Autodesk Inventor part; units mm, degrees
ref_plane "YZ Plane" through (0, 0, 0) normal (1, 0, 0) x (0, 1, 0)
ref_plane "XZ Plane" through (0, 0, 0) normal (0, 1, 0) x (-1, 0, 0)
ref_plane "XY Plane" through (0, 0, 0) normal (0, 0, 1) x (1, 0, 0)
sketch "Sketch1" plane through (0, 0, 0) normal (0, 0, 1) x (1, 0, 0)
  line L0 (0, 0) -> (25.4, 0)
  line L1 (25.4, 0) -> (25.4, -50.8)
  line L2 (25.4, -50.8) -> (0, -50.8)
  line L3 (0, -50.8) -> (0, 0)
  line L4 (3.175, -3.175) -> (22.225, -3.175)
  line L5 (22.225, -3.175) -> (22.225, -47.625)
  line L6 (22.225, -47.625) -> (3.175, -47.625)
  line L7 (3.175, -47.625) -> (3.175, -3.175)
  dimension "d0" = 25.4
  dimension "d1" = 50.8
  dimension "d2" = 19.05
  dimension "d3" = 44.45
  dimension "d4" = 3.175
  dimension "d5" = 3.175
extrude "Extrusion1" add sketch "Sketch1" along normal blind 76.2
sketch "Sketch2" plane through (0, -50.8, 0) normal (-1, 0, 0) x (0, 0, 1)
  line L0 (0, 0) -> (0, 50.8)
  line L1 (0, 0) -> (76.2, 0)
  point P0 (25.4, 20.6375)
  dimension "d8" = 20.6375
  dimension "d9" = 25.4
hole "Hole1" at (0, -30.1625, 25.4) direction (1, 0, 0) diameter 11.1125 end through all
properties part number "axle support 2x1" material "Aluminum 6061"
Input: part model. Units: mm. Frame: model coordinates. A direction names the side the tool comes from. Give positions to 0.01 mm unless a question says otherwise; leave off trailing zeros. Order: outer loops, then holes, each group sorted by start corner. A loop starts at its lowest first (then second) coordinate and runs counter-clockwise, first axis right, second up. Notation, with made-up numbers: M 87,41 L 136,41 A22 ccw 136,63 Z; hole C 53.5,81.5 d7. An arc over 180 degrees is marked long. One line per question, with ' | ' between items. Start each with the question number.
1. Section query C-C (y = -39.5). Return the cut outline in (x, z) (3 decimals), and give its area (3 significant figures).
2. Access query for faces 4 (the face through (1.61, -30.41, 19.85)), 5 (the face through (13, -47.625, 38)). Directions: +Z, -Z, +X, -X, +Y, -Y. A direction counts if a zero-diameter tool reaches every point of the face in a straight line with its end or side. Return the directions, or none.
3. First-contact query: pin 1 Ø10 at (y, z) = (-30.16, 25.4) entering from +X. Flat tip, straight axial feed; report the tip coordinate or a pass-through.
4. Pull-direction query (X, two-part tool) for faces 1 (the face through (13, -3.175, 38)), 2 (the face through (23.83, -30.41, 19.85)), 3 (the face through (0, -26, 38)); classes: released by +X, released by -X, zero draft, split by the parting line, or undercut.
5. Section query A-A (x = 9.5). Return the cut outline in (y, z) (3 decimals).
6. Material intervals for probe 1 along Y at (x, z) = (12.25, 50.5) (3 decimals); probe 2 along Y at (x, z) = (1.2, 25.4); probe 3 along X at (y, z) = (-17, 37) (3 decimals), sorted ascending. Write a range as [from, to].
7. Section query B-B (z = 25.4). Return the cut outline in (x, y) (3 decimals).
8. Section query D-D (y = -26). Return the cut outline in (x, z) (3 decimals), and give its area (3 significant figures).
Here are the results:
1) outline: M 0,0 L 3.175,0 L 3.175,76.2 L 0,76.2 Z; M 22.225,0 L 25.4,0 L 25.4,76.2 L 22.225,76.2 Z | area: 484 mm²
2) face 4: +X, -X | face 5: +Z, -Z
3) pin 1: through
4) face 1: undercut | face 2: zero draft | face 3: released by -X
5) outline: M -50.8,0 L -47.625,0 L -47.625,76.2 L -50.8,76.2 Z; M -3.175,0 L 0,0 L 0,76.2 L -3.175,76.2 Z
6) probe 1: [-50.8, -47.625], [-3.175, 0] | probe 2: [-50.8, -35.72], [-24.61, 0] | probe 3: [0, 3.175], [22.225, 25.4]
7) outline: M 0,-50.8 L 25.4,-50.8 L 25.4,-35.719 L 22.225,-35.719 L 22.225,-47.625 L 3.175,-47.625 L 3.175,-35.719 L 0,-35.719 Z; M 0,-24.606 L 3.175,-24.606 L 3.175,-3.175 L 22.225,-3.175 L 22.225,-24.606 L 25.4,-24.606 L 25.4,0 L 0,0 Z
8) outline: M 0,0 L 3.175,0 L 3.175,21.72 L 0,21.72 Z; M 0,29.08 L 3.175,29.08 L 3.175,76.2 L 0,76.2 Z; M 22.225,0 L 25.4,0 L 25.4,21.72 L 22.225,21.72 Z; M 22.225,29.08 L 25.4,29.08 L 25.4,76.2 L 22.225,76.2 Z | area: 437 mm²
